from build123d import *

# Parameters (mm, degrees)
SKETCH1_W           = 700
SKETCH1_H           = 150
BOSS_EXTRUDE1_DEPTH = 10
SKETCH2_W           = 680
SKETCH2_H           = 130
CUT_EXTRUDE1_DEPTH  = 10
SKETCH3_W           = 680
SKETCH3_H           = 10
BOSS_EXTRUDE2_DEPTH = 10
BOSS_EXTRUDE3_DEPTH = 10
SKETCH5_W           = 10
SKETCH5_H           = 10
BOSS_EXTRUDE4_DEPTH = 400


with BuildPart() as part:
    # Sketch1 → Boss-Extrude1 (new body)
    with BuildSketch(Plane(origin=(0, 0, 0), x_dir=(1, 0, 0), z_dir=(0, 1, 0))):
        Rectangle(SKETCH1_W, SKETCH1_H)
    extrude(amount=BOSS_EXTRUDE1_DEPTH)

    # Sketch2 → Cut-Extrude1 (cut)
    with BuildSketch(Plane(origin=(0, 10, 0), x_dir=(1, 0, 0), z_dir=(0, 1, 0))):
        Rectangle(SKETCH2_W, SKETCH2_H)
    extrude(amount=-CUT_EXTRUDE1_DEPTH, mode=Mode.SUBTRACT)

    # Sketch3 → Boss-Extrude2 (add)
    with BuildSketch(Plane(origin=(0, 10, 0), x_dir=(1, 0, 0), z_dir=(0, 1, 0))):
        with Locations((0, -5)):
            Rectangle(SKETCH3_W, SKETCH3_H)
    extrude(amount=-BOSS_EXTRUDE2_DEPTH)

    # Sketch4 → Boss-Extrude3 (add)
    with BuildSketch(Plane(origin=(0, 0, 0), x_dir=(1, 0, 0), z_dir=(0, 1, 0))):
        Polygon((5, 0), (0, 0), (7.5, 12.990381057), (12.5, 12.990381057), align=None)
        Polygon((140, 0), (147.5, 12.990381057), (152.5, 12.990381057), (145, 0), align=None)
        Polygon((140, 0), (132.5, 12.990381057), (127.5, 12.990381057), (135, 0), align=None)
        Polygon((0, 0), (-7.5, 12.990381057), (-12.5, 12.990381057), (-5, 0), align=None)
        Polygon((-140, 0), (-132.5, 12.990381057), (-127.5, 12.990381057), (-135, 0), align=None)
        Polygon((-140, 0), (-147.5, 12.990381057), (-152.5, 12.990381057), (-145, 0), align=None)
        Polygon((-280, 0), (-272.5, 12.990381057), (-267.5, 12.990381057), (-275, 0), align=None)
        Polygon((-280, 0), (-287.5, 12.990381057), (-292.5, 12.990381057), (-285, 0), align=None)
        Polygon((280, 0), (272.5, 12.990381057), (267.5, 12.990381057), (275, 0), align=None)
        Polygon((280, 0), (287.5, 12.990381057), (292.5, 12.990381057), (285, 0), align=None)
    extrude(amount=BOSS_EXTRUDE3_DEPTH)

    # Sketch5 → Boss-Extrude4 (add)
    with BuildSketch(Plane(origin=(0, 0, 0), x_dir=(1, 0, 0), z_dir=(0, 1, 0))):
        with Locations((-345, -5)):
            Rectangle(SKETCH5_W, SKETCH5_H)
        with Locations((345, -5)):
            Rectangle(SKETCH5_W, SKETCH5_H)
    extrude(amount=-BOSS_EXTRUDE4_DEPTH)


solid = part.part
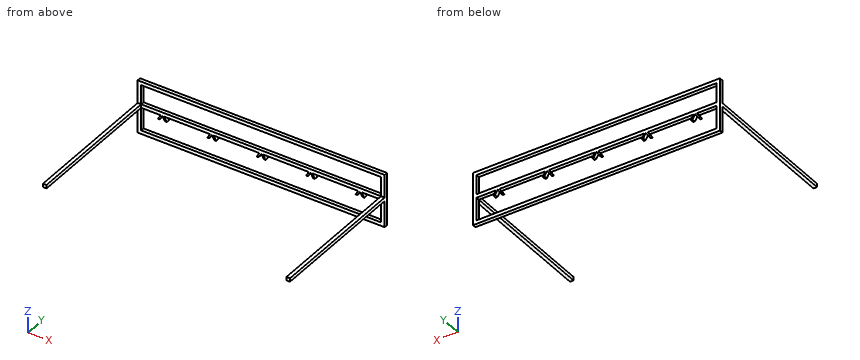
Model file for the job. Use its own axes, mm. Coordinates: 2 decimals unless noted, no trailing zeros. Write each loop counter-clockwise with the first axis right and the second up, starting at its lowest first coordinate (ties: lowest second). Pieces come first, ordered by that corner, then holes. Notation, with made-up numbers: (61, 63) -> (89, 63) arc R5 ccw to (89, 67) -> close; hole circle Ø4 at (44, 27.5). An arc over 180 degrees is marked (long way). One line per item, written item: value. Start each with the question number.
1) Slice it at A-A on y = -19. Write the cut outline in (x, z).
2) Slice it at B-B on x = 299.5. Write the cut outline in (y, z).
3) Probe probe 1 along Y at (x, z) = (-22, 6). List the from-to ranges inside material, lowest first.
4) Flat gauge pins, fed straight in: pin 1 Ø2 at (x, z) = (4.5, -6) entering from -Y; pin 2 Ø19.5 at (x, z) = (8.5, 46.5) entering from -Y. Where does each tip first touch, or does it go through?
Answers follow:
1. outline: (-350, 0) -> (-340, 0) -> (-340, 10) -> (-350, 10) -> close; (340, 0) -> (350, 0) -> (350, 10) -> (340, 10) -> close
2. outline: (0, -75) -> (10, -75) -> (10, -65) -> (0, -65) -> close; (0, 0) -> (10, 0) -> (10, 10) -> (0, 10) -> close; (0, 65) -> (10, 65) -> (10, 75) -> (0, 75) -> close
3. probe 1: 0 to 10
4. pin 1: y = 0
4. pin 2: through
